Part model, mm, in its own coordinate system. A direction names the side the tool comes from. Give positions to 0.01 mm unless a question says otherwise; leave off trailing zeros. Write each loop counter-clockwise with the first axis right and the second up, starting at its lowest first coordinate (ties: lowest second). Pieces come first, ordered by that corner, then holes. Notation, with made-up numbers: (37, 7.25) - (69, 7.25) arc R17 cw to (69, 23.25) - close; hole circle Ø3 at (51, 77.5). An arc over 180 degrees is marked (long way). Answer in a Markdown table with one row per item. Add a question column.
1. Pull direction Y, two halves, no side cores. Call faces 4 (the flat face through (-9, 15, -187)), 5 (the conical face through (4.759, 9.149, -0.313)), 6 (the conical face through (0, 1, -191)): released by +Y, released by -Y, zero draft, split by the parting line, or undercut.
2. Which spindle directions (+Z, -Z, +X, -X, +Y, -Y) get a long thin tool onto all of the face, cutting with end or side? Do faces 1 (the cylindrical face through (8.06, -12.65, -53.16)), 2 (the cylindrical face through (-19.98, -0.88, -184.49)), 3 (the flat face through (-10.5, -16.4, -181.9)). Say none if no direction does.
3. Drop flat-ended pins along their axis: pin 1 Ø3 at (y, z) = (-12.5, -80.5) entering from +X; pin 2 Ø5 at (y, z) = (5.5, -115) entering from +X; pin 3 Ø1 at (y, z) = (13.5, -110) entering from +X. Give the stop position or say it passes through.
4. Band-saw the part on A-A on z = -78.5. Write the cut outline in (x, y).
5. Probe line 1 along X through (y, z) = (9, -72.5); line 2 along Y through (x, z) = (-1.5, -154.5); line 3 along Y through (x, z) = (12.5, -173.5). List the from-to ranges inside material, lowest first.
```python
from build123d import *

# Parameters (mm, degrees)
CHAMFER_1_SIZE      = 5
SKETCH_4_R          = 20
SKETCH_4_R_2        = 19
CUT_EXTRUDE_1_DEPTH = 2
FILLET_1_R          = 0.3
CHAMFER_2_SIZE      = 1.5
SKETCH_9_R          = 25
SKETCH_9_R_2        = 20
CUT_EXTRUDE_4_DEPTH = 6
CHAMFER_3_SIZE      = 1.5


with BuildPart() as part:
    # Sketch 1 → Revolve 1 (revolve)
    with BuildSketch(Plane(origin=(0, 0, 0), x_dir=(0, 0, -1), z_dir=(1, 0, 0)), mode=Mode.PRIVATE) as revolve_1_sk:
        Polygon((0, 0), (0, 15), (100, 15), (100, 25), (147, 25), (147, 20), (187, 20), (187, 17), (195, 17), (195, 5), (190, 0), align=None)
    revolve(revolve_1_sk.sketch.rotate(Axis((0, 0, 0), (0, 0, -1)), 90), axis=Axis((0, 0, 0), (0, 0, -1)))

    # Chamfer 1
    chamfer_1_edges = [part.edges().sort_by_distance(p)[0] for p in [
        (-25, 0, -100),
        (-15, 0, 0),
        (-17, 0, -195),
    ]]
    chamfer(chamfer_1_edges, length=CHAMFER_1_SIZE)

    # Sketch 4 → Cut-Extrude 1 (cut)
    with BuildSketch(Plane(origin=(0, 0, -181.9), x_dir=(-1, 0, 0), z_dir=(0, 0, -1))):
        with Locations(Location((0, 0, 0), (0, 0, 180))):
            Circle(SKETCH_4_R)
        Circle(SKETCH_4_R_2, mode=Mode.SUBTRACT)
    extrude(amount=-CUT_EXTRUDE_1_DEPTH, mode=Mode.SUBTRACT)

    # Fillet 1
    fillet_1_edges = [part.edges().sort_by_distance(p)[0] for p in [
        (19, 0, -179.9),
        (19, 0, -181.9),
    ]]
    fillet(fillet_1_edges, radius=FILLET_1_R)

    # Chamfer 2
    chamfer_2_edges = [part.edges().sort_by_distance(p)[0] for p in [
        (-25, 0, -147),
    ]]
    chamfer(chamfer_2_edges, length=CHAMFER_2_SIZE)

    # Sketch 9 → Cut-Extrude 4 (cut)
    with BuildSketch(Plane(origin=(0, 0, -147), x_dir=(-1, 0, 0), z_dir=(0, 0, -1))):
        Circle(SKETCH_9_R)
        Circle(SKETCH_9_R_2, mode=Mode.SUBTRACT)
    extrude(amount=-CUT_EXTRUDE_4_DEPTH, mode=Mode.SUBTRACT)

    # Chamfer 3
    chamfer_3_edges = [part.edges().sort_by_distance(p)[0] for p in [
        (-25, 0, -141),
    ]]
    chamfer(chamfer_3_edges, length=CHAMFER_3_SIZE)


solid = part.part
```
Values:
| question | item | result |
|---|---|---|
| 1 | face 4 | zero draft |
| 1 | face 5 | split by the parting line |
| 1 | face 6 | undercut |
| 2 | face 1 | +Z |
| 2 | face 2 | -Z |
| 2 | face 3 | none |
| 3 | pin 1 | stops at x = 10.2 |
| 3 | pin 2 | stops at x = 24.82 |
| 3 | pin 3 | stops at x = 21.35 |
| 4 | outline | circle Ø30 at (0, 0) |
| 5 | line 1 | x = -12 to 12 |
| 5 | line 2 | y = -19.94 to 19.94 |
| 5 | line 3 | y = -15.61 to 15.61 |
